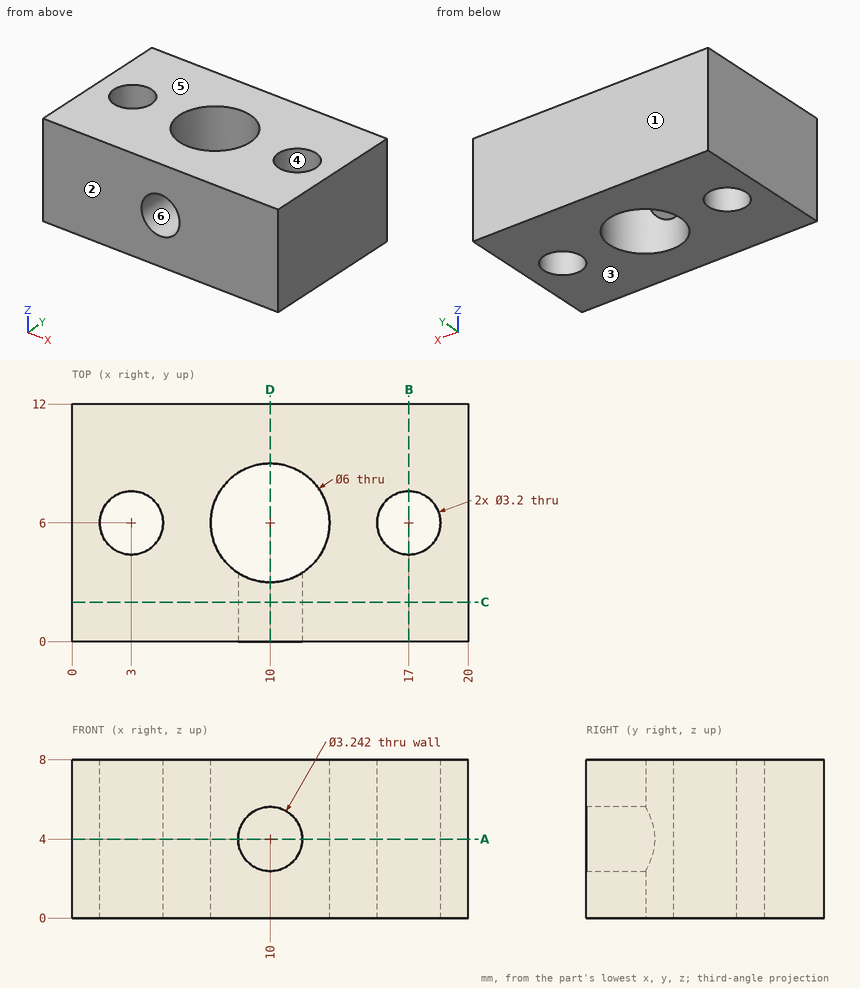
Design review of the part shown in the three views and the two pictorial views. Dimensions are in mm from the part's minimum x, y and z. A direction names the side the tool comes from. Round coordinates to 2 decimals unless told otherwise and drop trailing zeros. Write each loop counter-clockwise with the first axis right and the second up, starting at its lowest first coordinate (ties: lowest second). Pieces come first, ordered by that corner, then holes. Notation, with made-up numbers: (-5, 49.25) -> (20, 49.25) arc R12 ccw to (20, 53.25) -> close; hole circle Ø10 at (41, 35). An arc over 180 degrees is marked (long way). Use one line per item in the form item = value.
1) To check wall thickness, follow L1, parallel to X at y = 6, z = 2; L2, parallel to X at y = 1.75, z = 4; L3, parallel to Y at x = 10, z = 6.25. State the ranges of each line that lie inside material, in increasing order. Write a range as from..to.
Found:
L1 = 0..1.4, 4.6..7, 13..15.4, 18.6..20
L2 = 0..8.38, 11.62..20
L3 = 0..3, 9..12
2) Take a section at B-B, the plane x = 17. Write out the cut boundary in (y, z).
Found:
outline = (0, 0) -> (4.4, 0) -> (4.4, 8) -> (0, 8) -> close; (7.6, 0) -> (12, 0) -> (12, 8) -> (7.6, 8) -> close
3) Clearance check with flat-ended pins moving along their axes: pin 1 (3 mm diameter, centred on x = 10, z = 4, fed in from -Y); pin 2 (1.5 mm diameter, centred on y = 7.5, z = 3.5, fed in from -X). State where each tip first meets the part, or that it passes through.
Found:
pin_1 = 8.6
pin_2 = 0
4) Tool access review of the marked faces 5 and 6: name each direction out of +Z, -Z, +X, -X, +Y, -Y from which nothing blocks a thin tool from reaching the whole face with its end or side.
Found:
face_5 = +Z, +X, -X, +Y, -Y
face_6 = -Y
5) Take a section at C-C, the plane y = 2. Write out the cut boundary in (x, z).
Found:
outline = (0, 0) -> (20, 0) -> (20, 8) -> (0, 8) -> close; hole circle Ø3.24 at (10, 4)
6) Take a section at A-A, the plane z = 4. Write out the cut boundary in (x, y), and give its area (3 significant figures).
Found:
outline = (0, 0) -> (8.38, 0) -> (8.38, 3.48) arc R3 cw (long way) to (11.62, 3.48) -> (11.62, 0) -> (20, 0) -> (20, 12) -> (0, 12) -> close; hole circle Ø3.2 at (3, 6); hole circle Ø3.2 at (17, 6)
area = 185 mm2
7) Mouldability with a two-part tool opening along Y and no side actions: class the marked faces 1, 2, 3 and 4 as +Y half, -Y half, draft (parallel to the pull), parting line (faces both ways), or undercut.
Found:
face_1 = +Y half
face_2 = -Y half
face_3 = draft
face_4 = undercut
8) Take a section at D-D, the plane x = 10. Write out the cut boundary in (y, z).
Found:
outline = (0, 0) -> (3, 0) -> (3, 2.38) -> (0, 2.38) -> close; (0, 5.62) -> (3, 5.62) -> (3, 8) -> (0, 8) -> close; (9, 0) -> (12, 0) -> (12, 8) -> (9, 8) -> close
